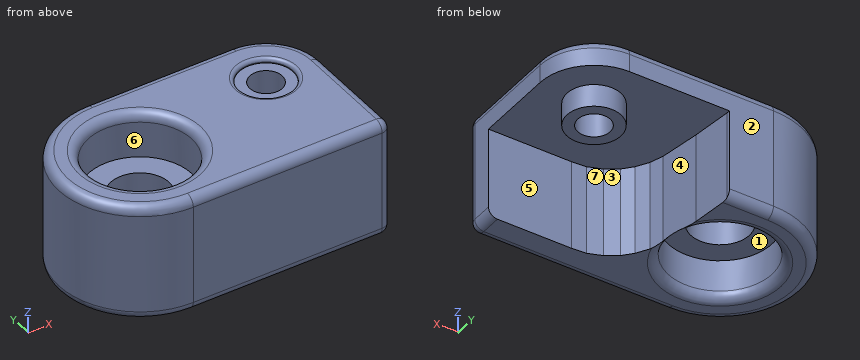
from build123d import *

# Parameters (mm, degrees)
CYLINDER114_R     = 1.8
CYLINDER114_DEPTH = 7
CYLINDER115_R     = 3
CYLINDER115_DEPTH = 7
PAD_DEPTH         = 30
BOX002_W          = 10
BOX002_H          = 10
BOX002_DEPTH      = 10
BOX003_W          = 17
BOX003_H          = 10
BOX003_DEPTH      = 10
CYLINDER018_R     = 5.75
CYLINDER018_DEPTH = 10
CYLINDER017_R     = 3.25
CYLINDER017_DEPTH = 10
CYLINDER113_R     = 5.75
CYLINDER113_DEPTH = 10
CYLINDER112_R     = 3.25
CYLINDER112_DEPTH = 10
BOX_W             = 22
BOX_H             = 18
BOX_DEPTH         = 13
CYLINDER111_R     = 9
CYLINDER111_DEPTH = 13
FILLET038_R       = 6
FILLET001_R       = 1
FILLET002_R       = 1
FILLET003_R       = 1
CYLINDER019_R     = 3
CYLINDER019_DEPTH = 3
FILLET004_R       = 0.4


with BuildPart() as m3cut:
    # Cylinder114 → Cylinder114 (new body)
    with BuildSketch(Plane(origin=(-4.5, -22, 62.5), x_dir=(1, 0, 0), z_dir=(0, 0, 1))):
        Circle(CYLINDER114_R)
    extrude(amount=CYLINDER114_DEPTH)


with BuildPart() as fusion009:
    # Cylinder115 → Cylinder115 (new body)
    with BuildSketch(Plane(origin=(-4.5, -22, 67.5), x_dir=(1, 0, 0), z_dir=(0, 0, 1))):
        Circle(CYLINDER115_R)
    extrude(amount=CYLINDER115_DEPTH)

    # Fusion009: union m3Cut
    add(m3cut.part)


with BuildPart() as body012:
    # Sketch066 → Pad (new body)
    with BuildSketch(Plane.XY):
        Polygon((-15.594093, -16.374565), (-15.071085, -20.857502), (-14.364655, -25.305099), (-13.862565, -26.78348), (-13.081532, -28.094496), (-12.161032, -29.126572), (-10.822123, -30.019178), (-9.315848, -30.577057), (-7.725893, -30.688633), (7.476312, -30.688633), (-15.876865, 6.281797), (-15.876865, -11.843776), align=None)
    extrude(amount=PAD_DEPTH)

    # Box002 → Box002 (join)
    with BuildSketch(Plane.XY):
        with Locations((5, 5)):
            Rectangle(BOX002_W, BOX002_H)
    extrude(amount=BOX002_DEPTH)


with BuildPart() as body012_1:
    # Body placement: moved
    add(body012.part.moved(Location((0, 0, 35))))


with BuildPart() as firstcuts:
    # Box003 → Box003 (new body)
    with BuildSketch(Plane(origin=(-10, -24, 55), x_dir=(1, 0, 0), z_dir=(0, 0, 1))):
        with Locations((8.5, 5)):
            Rectangle(BOX003_W, BOX003_H)
    extrude(amount=BOX003_DEPTH)

    # Fusion007: union Body012
    add(body012_1.part)


with BuildPart() as obj1:
    # Cylinder018 → Cylinder018 (new body)
    with BuildSketch(Plane(origin=(-23, 0, 69), x_dir=(1, 0, 0), z_dir=(0, 0, 1))):
        Circle(CYLINDER018_R)
    extrude(amount=CYLINDER018_DEPTH)


with BuildPart() as fusion065:
    # Cylinder017 → Cylinder017 (new body)
    with BuildSketch(Plane(origin=(-23, 0, 65), x_dir=(1, 0, 0), z_dir=(0, 0, 1))):
        Circle(CYLINDER017_R)
    extrude(amount=CYLINDER017_DEPTH)

    # Fusion065: union obj1
    add(obj1.part)


with BuildPart() as fusion065_1:
    # Fusion065 placement: moved
    add(fusion065.part.moved(Location((2.5, -25, -19.5))))


with BuildPart() as obj2:
    # Cylinder113 → Cylinder113 (new body)
    with BuildSketch(Plane(origin=(-23, 0, 69), x_dir=(1, 0, 0), z_dir=(0, 0, 1))):
        Circle(CYLINDER113_R)
    extrude(amount=CYLINDER113_DEPTH)


with BuildPart() as antennacuts:
    # Cylinder112 → Cylinder112 (new body)
    with BuildSketch(Plane(origin=(-23, 0, 65), x_dir=(1, 0, 0), z_dir=(0, 0, 1))):
        Circle(CYLINDER112_R)
    extrude(amount=CYLINDER112_DEPTH)

    # Fusion064: union obj2
    add(obj2.part)


with BuildPart() as antennacuts_1:
    # Fusion064 placement: moved
    add(antennacuts.part.moved(Location((2.5, -25, -6))))

    # Fusion006: union Fusion065
    add(fusion065_1.part)


with BuildPart() as cube:
    # Box → Box (new body)
    with BuildSketch(Plane(origin=(-20.5, -34, 56), x_dir=(1, 0, 0), z_dir=(0, 0, 1))):
        with Locations((11, 9)):
            Rectangle(BOX_W, BOX_H)
    extrude(amount=BOX_DEPTH)


with BuildPart() as cut001:
    # Cylinder111 → Cylinder111 (new body)
    with BuildSketch(Plane(origin=(-20.5, -25, 56), x_dir=(1, 0, 0), z_dir=(0, 0, 1))):
        Circle(CYLINDER111_R)
    extrude(amount=CYLINDER111_DEPTH)

    # Fusion063: union Cube
    add(cube.part)


with BuildPart() as cut001_1:
    # Fusion063 placement: moved
    add(cut001.part.moved(Location((0, 0, -1))))

    # Fillet038
    fillet038_edges = [cut001_1.edges().sort_by_distance(p)[0] for p in [
        (1.5, -16, 61.5),
    ]]
    fillet(fillet038_edges, radius=FILLET038_R)

    # Fillet001
    fillet001_edges = [cut001_1.edges().sort_by_distance(p)[0] for p in [
        (-12.5, -16, 55),
        (1.5, -28, 55),
        (-14.136039, -31.363961, 55),
        (-20.5, -16, 61.5),
        (1.5, -28, 68),
        (1.5, -34, 61.5),
        (-9.5, -34, 68),
        (-29.5, -25, 55),
        (-29.5, -25, 68),
    ]]
    fillet(fillet001_edges, radius=FILLET001_R)

    # Cut029: cut antennaCuts
    add(antennacuts_1.part, mode=Mode.SUBTRACT)

    # Fillet002
    fillet002_edges = [cut001_1.edges().sort_by_distance(p)[0] for p in [
        (-16.434136, -29.065864, 68),
        (-16.434136, -20.934136, 68),
    ]]
    fillet(fillet002_edges, radius=FILLET002_R)

    # Fillet003
    fillet003_edges = [cut001_1.edges().sort_by_distance(p)[0] for p in [
        (0.5, -27.5, 55),
        (1.207107, -33, 55.292893),
        (-26.25, -25, 55),
    ]]
    fillet(fillet003_edges, radius=FILLET003_R)

    # Cut001: cut firstCuts
    add(firstcuts.part, mode=Mode.SUBTRACT)


with BuildPart() as antennaholder:
    # Cylinder019 → Cylinder019 (new body)
    with BuildSketch(Plane(origin=(-4.5, -22, 62.5), x_dir=(1, 0, 0), z_dir=(0, 0, 1))):
        Circle(CYLINDER019_R)
    extrude(amount=CYLINDER019_DEPTH)

    # Fusion008: union Cut001
    add(cut001_1.part)

    # Cut002: cut Fusion009
    add(fusion009.part, mode=Mode.SUBTRACT)


with BuildPart() as antennaholder_1:
    # Cut002 placement: moved
    add(antennaholder.part.moved(Location((74.8, 0, -176.8))))

    # Fillet004
    fillet004_edges = [antennaholder_1.edges().sort_by_distance(p)[0] for p in [
        (67.3, -22, -108.8),
    ]]
    fillet(fillet004_edges, radius=FILLET004_R)


with BuildPart() as antennaholder_2:
    # Fillet004 placement: moved
    add(antennaholder_1.part.moved(Location((400, 0, -268.2))))


solid = antennaholder_2.part
Could you check a few things on this model? Use its own coordinates, in mm. Face numbers are marked on the shaded views. A direction names the side the tool comes from. Give positions to 0.01 mm unless a question says otherwise; leave off trailing zeros. Loops run counter-clockwise (first coordinate to the right, second up) from the corner with the lowest first, then second, coordinate; pieces in that order, holes last. Notation, with made-up numbers: (88.25, 60) -> (97.25, 60) arc R15 ccw to (97.25, 77) -> close; hole circle Ø4 at (41, -11.75). An arc over 180 degrees is marked (long way). Answer as CSV lines item,"result". Start each with the question number.
(1) I'm going to push flat-ended pins straight in: pin 1 Ø6 at (x, y) = (453.5, -28.5) entering from +Z; pin 2 Ø3.5 at (x, y) = (456, -23) entering from -Z; pin 3 Ø3.5 at (x, y) = (470.3, -22) entering from -Z; pin 4 Ø4.5 at (x, y) = (465, -19.5) entering from -Z. Where does each tip first touch, or does it pass through?
(2) If we section it at B-B on z = -388.5: Write out the boundary of the cut face in (x, y).
(3) Which directions (+Z, -Z, +X, -X, +Y, -Y) give clear straight access to the entire face, cutting with the end or side of a thin tool? Please do the marked faces 4, 5, 6 and 7.
(4) We'd pull the mould along X, two halves only. Please class the marked faces 1, 2 and 3: released by +X, released by -X, zero draft, split by the parting line, or undercut.
(5) If we section it at A-A on z = -384.5: Write out the boundary of the cut face in (x, y).
(6) I need wall thicknesses on probe 1 along Y at (x, z) = (470.3, -381.3); probe 2 along X at (y, z) = (-25, -379.1); probe 3 along Y at (x, z) = (454.3, -380.35). Which ranges of each line are inside material? Lowest first, please.
(7) If we section it at C-C on x = 463: Write out the boundary of the cut face in (y, z).
Computed:
1,pin 1,"stops at z = -377.01"
1,pin 2,"stops at z = -385.5"
1,pin 3,"passes through"
1,pin 4,"stops at z = -380"
2,outline,"(454.3, -34) -> (475.3, -34) arc R1 ccw to (476.3, -33) -> (476.3, -30.69) -> (467.07, -30.69) -> (465.48, -30.58) -> (463.98, -30.02) -> (462.64, -29.13) -> (461.72, -28.09) -> (460.94, -26.78) -> (460.44, -25.31) -> (459.73, -20.86) -> (459.21, -16.37) -> (459.18, -16) -> (454.3, -16) arc R9 ccw to start; hole circle Ø11.5 at (454.3, -25)"
3,face 4,"-Z, +Y"
3,face 5,"-Z, +X"
3,face 6,"+Z"
3,face 7,"-Z, +X, +Y"
4,face 1,"undercut"
4,face 2,"zero draft"
4,face 3,"released by +X"
5,outline,"(454.3, -34) -> (475.3, -34) arc R1 ccw to (476.3, -33) -> (476.3, -30.69) -> (467.07, -30.69) -> (465.48, -30.58) -> (463.98, -30.02) -> (462.64, -29.13) -> (461.72, -28.09) -> (460.94, -26.78) -> (460.44, -25.31) -> (459.73, -20.86) -> (459.21, -16.37) -> (459.18, -16) -> (454.3, -16) arc R9 ccw to start; hole circle Ø6.5 at (454.3, -25)"
6,probe 1,"y = -34 to -30.69, -25 to -23.8, -20.2 to -19"
6,probe 2,"x = 445.3 to 448.55, 460.05 to 476.3"
6,probe 3,"y = -34 to -30.75, -19.25 to -16"
7,outline,"(-34, -389) arc R1 ccw to (-33, -390) -> (-29.37, -390) -> (-29.37, -380) -> (-16, -380) -> (-16, -378) arc R1 ccw to (-17, -377) -> (-33, -377) arc R1 ccw to (-34, -378) -> close"
